Could you check a few things on this model? Use its own coordinates, in mm. A direction names the side the tool comes from. Round coordinates to 2 decimals unless told otherwise and drop trailing zeros. Loops run counter-clockwise (first coordinate to the right, second up) from the corner with the lowest first, then second, coordinate; pieces in that order, holes last. Notation, with made-up numbers: (-15, 43.25) - (13, 43.25) arc R11 ccw to (13, 60.25) - close; hole circle Ø3 at (29, -26.75). An arc over 180 degrees is marked (long way). Answer as CSV lines item,"result". Start each with the question number.
1) Suppose I cut it at C-C, the plane x = 74. Write out the boundary of the cut face in (y, z).
2) Suppose I cut it at A-A, the plane z = 5. Write out the boundary of the cut face in (x, y).
3) We'd pull the mould along X, two halves only. Please class faces 4 (the face through (99, 10, -60)), 5 (the face through (-85, 18, 1)), 6 (the face through (97, 6, -46)): pulls with the +X half, pulls with the -X half, needs draft (parallel to the pull), parting line crosses it, or undercut.
4) Please list where these lines run through material, in increasing order: line 1 along Z through (x, y) = (-73, 20); line 2 along X through (y, z) = (20.5, 24.5); line 3 along X through (y, z) = (9, 2.5).
5) I'm going to push flat-ended pins straight in: pin 1 Ø8.5 at (x, y) = (-73, 14) entering from -Z; pin 2 Ø5 at (y, z) = (19, -38) entering from +X; pin 3 Ø3 at (x, y) = (6, 30) entering from -Z; pin 4 Ø11 at (y, z) = (23, 8) entering from +X. Where does each tip first touch, or does it pass through?
6) Suppose I cut it at D-D, the plane x = -39.5. Write out the boundary of the cut face in (y, z).
7) Which directions (+Z, -Z, +X, -X, +Y, -Y) give clear straight access to the entire face, cutting with the end or side of a thin tool? Please do faces 1 (the face through (82, 23.4, 16.9)), 2 (the face through (0, 37, 29)), 3 (the face through (61, 20, 23)).
8) Suppose I cut it at B-B, the plane y = 9. Write out the boundary of the cut face in (x, z).
Autodesk Inventor part; units mm, degrees
ref_plane "YZ Plane" through (0, 0, 0) normal (1, 0, 0) x (0, 1, 0)
ref_plane "XZ Plane" through (0, 0, 0) normal (0, 1, 0) x (-1, 0, 0)
ref_plane "XY Plane" through (0, 0, 0) normal (0, 0, 1) x (1, 0, 0)
sketch "Sketch1" plane through (0, 0, 0) normal (0, 1, 0) x (-1, 0, 0)
  line L0 (85, 30) -> (-85, 30)
  line L1 (-85, 30) -> (-85, -30)
  line L2 (-85, -30) -> (85, -30)
  line L3 (85, -30) -> (85, 30)
  line L4 (85, 30) -> (-85, -30) construction
  line L5 (-85, 30) -> (85, -30) construction
  line L6 (-85, -30) -> (-100, -30)
  line L7 (-100, -30) -> (-100, -27)
  line L8 (-100, -27) -> (-85, -27)
  line L9 (0, -42) -> (0, 42)
  line L10 (85, -30) -> (100, -30)
  line L11 (100, -30) -> (100, -27)
  line L12 (100, -27) -> (85, -27)
  point P0 (0, 0)
  point P1 (85, -27)
  dimension "d0" = 170
  dimension "d1" = 60
  dimension "d32" = 15
  dimension "d33" = 3
extrude "Extrusion1" add sketch "Sketch1" along normal blind 3
sketch "Sketch2" plane through (0, 3, 0) normal (0, 1, 0) x (1, 0, 0)
  line L0 (-85, 27) -> (-85, -30)
  line L1 (-85, -30) -> (85, -30)
  line L2 (85, -30) -> (85, 27)
  line L3 (100, 30) -> (-100, 30)
  line L4 (-100, 30) -> (-100, 27)
  line L5 (-100, 27) -> (-85, 27)
  line L6 (85, 27) -> (100, 27)
  line L7 (100, 27) -> (100, 30)
  line L8 (82, -27) -> (-82, -27)
  line L9 (-82, -27) -> (-82, 27)
  line L10 (-82, 27) -> (82, 27)
  line L11 (82, 27) -> (82, -27)
  line L12 (82, -27) -> (-82, 27) construction
  line L13 (-82, -27) -> (82, 27) construction
  point P0 (0, 0)
  dimension "d36" = 164
  dimension "d37" = 54
extrude "Extrusion2" add sketch "Sketch2" along normal blind 34
sketch "Sketch7" plane through (-82, 3, 27) normal (1, 0, 0) x (0, 0, -1)
  circle A0 centre (10, 17) radius 8
  line L0 (54, -3) -> (-3, -3)
  circle A1 centre (10, 17) radius 10
  line L1 (0, 17) -> (0, 0)
  line L2 (0, 17) -> (20, 17)
  line L3 (20, 17) -> (20, 0)
  line L4 (-3, -3) -> (-3, 34)
  line L5 (0, 0) -> (20, 0)
  line L6 (10, 27) -> (0, 27)
  line L7 (0, 0) -> (0, 34)
  line L8 (0, 17) -> (0, 27)
  point P0 (27, -3)
  point P1 (57, -3)
  dimension "d17" = 16
  dimension "d18" = 20
  dimension "d20" = 2
  dimension "d40" = 20
  dimension "d62" = 10
extrude "Extrusion5" add sketch "Sketch7" along normal blind 11.25 contours L2 A1 A0 | A0 L2 A1 | L3 L5 L1 A1 | L7 L6 A1
sketch "Sketch8" plane through (-70.75, 3, 27) normal (1, 0, 0) x (0, 0, -1)
  arc A0 (20, 17) -> (10, 27) centre (10, 17) ccw
  circle A1 centre (10, 17) radius 8
  line L0 (0, 0) -> (0, 27)
  line L1 (20, 0) -> (0, 0)
  line L2 (20, 0) -> (20, 17)
  circle A2 centre (10, 17) radius 7.75
  line L3 (10, 27) -> (0, 27)
  line L4 (0, 0) -> (0, 27)
  line L5 (4, 12.0946) -> (4, 22.2915)
  line L6 (10, 27) -> (0, 27)
  line L7 (16, 12.0946) -> (16, 22.2915)
  line L8 (16, 22.2915) -> (18.4853, 22.2915)
  arc A3 (20, 17) -> (10, 27) centre (10, 17) ccw
  line L9 (4, 22.2915) -> (0, 22.2915)
  point P0 (27, -3)
  point P1 (4, 27)
  point P2 (18.4853, 22.2915)
  point P3 (4, 21.9054)
  point P4 (16, 21.9054)
  dimension "d55" = 15.5
  dimension "d63" = 12
  dimension "d64" = 6
extrude "Extrusion6" add sketch "Sketch8" along normal blind 20 contours L2 L1 L0 L9 A1 L8 A0 | A1 L5 A2 L7 | A2 L7 | L5 A2 picked at (9.114, 9.2488)
sketch "Sketch9" plane through (-82, 20, 17) normal (1, 0, 0) x (0, 0, -1)
  circle A0 centre (0, 0) radius 3
  line L0 (44, -20) -> (-13, -20)
  line L1 (-13, -20) -> (-13, 17)
  point P0 (17, -20)
  point P1 (47, -20)
  dimension "d27" = 6
  dimension "d28" = 20
  dimension "d41" = 13
extrude "Extrusion7" cut sketch "Sketch9" against normal up to surface (3 mm away)
mirror "Mirror2" about plane through (0, 0, 0) normal (1, 0, 0) of "Extrusion7", "Extrusion6", "Extrusion5"
sketch "Sketch4" plane through (-87, 3, -27) normal (0, 0, 1) x (1, 0, 0)
  line L0 (87, 34) -> (107, 34)
  line L1 (87, 34) -> (67, 34)
  line L2 (67, 34) -> (67, 0)
  line L3 (107, 34) -> (107, 0)
  line L4 (107, 0) -> (67, 0)
  line L5 (5, 0) -> (5, 34)
  line L6 (5, 34) -> (169, 34)
  line L7 (67, 12) -> (70, 12)
  line L8 (70, 12) -> (70, 0)
  line L9 (107, 12) -> (104, 12)
  line L10 (104, 12) -> (104, 0)
  point P0 (87, -3)
  dimension "d13" = 20
  dimension "d14" = 20
  dimension "d42" = 82
  dimension "d43" = 34
  dimension "WeaponMountThickness" = 3
  dimension "WeaponMountSlot" = 12
extrude "Extrusion9" cut sketch "Sketch4" against normal up to surface (3 mm away) contours L0 L3 L9 L10 L4 L8 L7 L2 L1
sketch "Sketch13" plane through (100, 0, -27) normal (1, 0, 0) x (0, 0, -1)
  line L0 (0, 0) -> (3, 0)
  line L1 (3, 0) -> (3, 20)
  line L2 (0, 0) -> (0, 37)
  line L3 (3, 20) -> (63, 0)
  line L4 (63, 0) -> (3, 0)
  point P0 (-27, 0)
  dimension "d60" = 60
  dimension "d61" = 20
extrude "Extrusion11" add sketch "Sketch13" against normal blind 3
mirror "Mirror4" about plane through (0, 0, 0) normal (1, 0, 0) of "Extrusion11"
sketch "Sketch14" plane through (0, 3, 0) normal (0, 1, 0) x (1, 0, 0)
  point P0 (0, 0)
equation "\"d0\" = Width"
equation "\"d1\" = Length"
equation "\"d32\" = -0.5 * Width + 0.5 * FullWidth"
equation "\"d33\" = SideWallThickness"
equation "\"d2\" = BaseWallThickness"
equation "\"d36\" = Width - 2 * SideWallThickness"
equation "\"d37\" = Length - 2 * SideWallThickness"
equation "\"d5\" = Height - 2 * BaseWallThickness"
equation "\"d18\" = DriveMotorHeight"
equation "\"d20\" = DriveMotorMountThickness"
equation "\"d28\" = DriveMotorHeight"
equation "\"d13\" = 0.5 * WeaponSlotWidth"
equation "\"d14\" = 0.5 * WeaponSlotWidth"
equation "\"d42\" = 0.5 * Width - SideWallThickness"
equation "\"d43\" = Height - 2 * BaseWallThickness"
equation "\"d60\" = WedgeLength"
equation "\"d61\" = WedgeHeight"
equation "\"d53\" = SideWallThickness"
equation "\"SideWallThickness\" = 3"
equation "\"BaseWallThickness\" = 3"
equation "\"Width\" = 170"
equation "\"Length\" = 60"
equation "\"DriveMotorHeight\" = 20"
equation "\"DriveMotorMountThickness\" = 2"
equation "\"WedgeLength\" = 60"
equation "\"WedgeHeight\" = 20"
properties part number "BodyV2" material "Thermoplastic Resin"
Filled sheet:
1,outline,"(0, -30) - (37, -30) - (37, -27) - (3, -27) - (3, 7) - (20, 7) arc R10 ccw to (30, 17) - (30, 27) - (37, 27) - (37, 30) - (0, 30) - close; hole circle Ø16 at (20, 17)"
2,outline,"(-85, 0) - (85, 0) - (85, 37) - (82, 37) - (82, 3) - (-82, 3) - (-82, 37) - (-85, 37) - close"
3,face 4,"needs draft"
3,face 5,"pulls with the -X half"
3,face 6,"undercut"
4,line 1,"-30 to -27, 7 to 9, 25 to 30"
4,line 2,"-85 to -82, -70.75 to -50.75, 50.75 to 70.75, 82 to 85"
4,line 3,"-85 to -82, 82 to 85"
5,pin 1,"z = -30"
5,pin 2,"x = 100"
5,pin 3,"z = 27"
5,pin 4,"x = 85"
6,outline,"(0, -30) - (37, -30) - (37, -27) - (3, -27) - (3, 27) - (37, 27) - (37, 30) - (0, 30) - close"
7,face 1,"none"
7,face 2,"+Z, -Z, +X, -X, +Y"
7,face 3,"+Y"
8,outline,"(-100, -63) - (-97, -63) - (-97, -30) - (-17, -30) - (-17, -27) - (-82, -27) - (-82, 7) - (-50.75, 7) - (-50.75, 27) - (50.75, 27) - (50.75, 7) - (82, 7) - (82, -27) - (17, -27) - (17, -30) - (97, -30) - (97, -63) - (100, -63) - (100, -27) - (85, -27) - (85, 30) - (-85, 30) - (-85, -27) - (-100, -27) - close"
